Build history of the part. All positions in model axes, mm. Face numbers are marked on the shaded views. A direction names the side the tool comes from. Give positions to 0.01 mm unless a question says otherwise; leave off trailing zeros. Write each loop counter-clockwise with the first axis right and the second up, starting at its lowest first coordinate (ties: lowest second). Pieces come first, ordered by that corner, then holes. Notation, with made-up numbers: (-6.5, -12) -> (35.5, -12) arc R4 cw to (35.5, -6) -> close; hole circle Ø6 at (22.25, 42). An arc over 180 degrees is marked (long way). One line per question, with ' | ' between items. Start each with the question number.
(1) Band-saw the part on D-D, the plane z = -4.25. Give the cut face in (x, y), and give its area (3 significant figures).
(2) Band-saw the part on C-C, the plane y = 11.75. Give the cut face in (x, z).
(3) Tool access for the marked faces 5 and 6: list every direction of +Z, -Z, +X, -X, +Y, -Y with a clear straight run to the whole face (end or side of a thin tool).
(4) Band-saw the part on A-A, the plane x = -7.5. Give the cut face in (y, z).
(5) Pin check, flat tip, straight feed: P1, Ø3, axis at x = 6.5, z = 6, coming from the +Y side. Stop position of the tip, or through.
(6) Drill centre lines: probe 1 along X at (y, z) = (15.5, 6.25); probe 2 along X at (y, z) = (4, -6.75); probe 3 along Z at (x, y) = (-6.25, 4.5). Where is each one in solid material? Low to high. Write a range as from..to.
(7) Pull direction X, two halves, no side cores. Call the marked faces 1, 2, 3 and 4: released by +X, released by -X, zero draft, split by the parting line, or undercut.
(8) Band-saw the part on B-B, the plane z = -7.5. Give the cut face in (x, y).
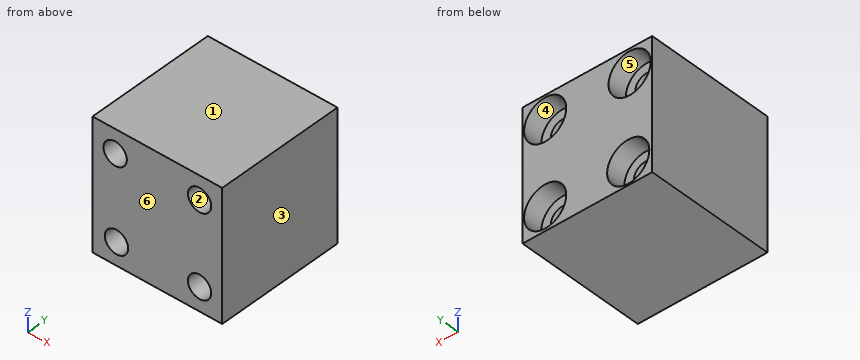
from build123d import *

# Parameters (mm, degrees)
ESBO_O1_W                         = 20
ESBO_O1_H                         = 20
RESSALTO_EXTRUS_O1_DEPTH          = 20
REBAIXO_PARA_SHCS_M32_D           = 3.6
REBAIXO_PARA_SHCS_M32_CBORE_D     = 6.5
REBAIXO_PARA_SHCS_M32_CBORE_DEPTH = 3


with BuildPart() as part:
    # Esboço1 → Ressalto-extrusão1 (new body)
    with BuildSketch(Plane(origin=(0, 0, 0), x_dir=(1, 0, 0), z_dir=(0, 1, 0))):
        Rectangle(ESBO_O1_W, ESBO_O1_H)
    extrude(amount=RESSALTO_EXTRUS_O1_DEPTH)

    # Rebaixo para SHCS M32 (through all)
    with Locations(Plane(origin=(-6.303242204, 20, -6.525555725), x_dir=(0, 0, 1), z_dir=(0, 1, 0))):
        with Locations((0, 0), (0.156927192, 12.815720663), (12.92033879, 12.815720663), (12.894184258, -0.209236255)):
            CounterBoreHole(REBAIXO_PARA_SHCS_M32_D / 2, REBAIXO_PARA_SHCS_M32_CBORE_D / 2, REBAIXO_PARA_SHCS_M32_CBORE_DEPTH)


solid = part.part
Results:
1) outline: (-10, 0) -> (10, 0) -> (10, 20) -> (8.98, 20) -> (8.98, 17) -> (4.05, 17) -> (4.05, 20) -> (-3.98, 20) -> (-3.98, 17) -> (-8.62, 17) -> (-8.62, 20) -> (-10, 20) -> close | area: 371 mm²
2) outline: (-10, -10) -> (10, -10) -> (10, 10) -> (-10, 10) -> close; hole circle Ø3.6 at (-6.51, 6.37); hole circle Ø3.6 at (-6.3, -6.53); hole circle Ø3.6 at (6.51, -6.37); hole circle Ø3.6 at (6.51, 6.39)
3) face 5: +Y | face 6: +Z, -Z, +X, -X, -Y
4) outline: (0, -10) -> (20, -10) -> (20, -9.55) -> (17, -9.55) -> (17, -7.87) -> (0, -7.87) -> close; (0, -5.18) -> (17, -5.18) -> (17, -3.5) -> (20, -3.5) -> (20, 3.27) -> (17, 3.27) -> (17, 4.86) -> (0, 4.86) -> close; (0, 7.87) -> (17, 7.87) -> (17, 9.46) -> (20, 9.46) -> (20, 10) -> (0, 10) -> close
5) P1: stops at y = 17
6) probe 1: x = -10..-8.31, -4.72..4.72, 8.31..10 | probe 2: x = -10..-8.09, -4.52..4.75, 8.27..10 | probe 3: z = -10..-8.32, -4.73..4.59, 8.15..10
7) face 1: zero draft | face 2: undercut | face 3: released by +X | face 4: undercut
8) outline: (-10, 0) -> (-7.82, 0) -> (-7.82, 17) -> (-9.4, 17) -> (-9.4, 20) -> (-10, 20) -> close; (-4.79, 0) -> (5.11, 0) -> (5.11, 17) -> (3.47, 17) -> (3.47, 20) -> (-3.2, 20) -> (-3.2, 17) -> (-4.79, 17) -> close; (7.91, 0) -> (10, 0) -> (10, 20) -> (9.56, 20) -> (9.56, 17) -> (7.91, 17) -> close
